Model file for the job. Use its own axes, mm. Give positions to 0.01 mm unless a question says otherwise; leave off trailing zeros. Order: outer loops, then holes, each group sorted by start corner. A loop starts at its lowest first (then second) coordinate and runs counter-clockwise, first axis right, second up. Notation, with made-up numbers: (8, 57.5) -> (20, 57.5) arc R29 ccw to (20, 88.5) -> close; hole circle Ø9 at (24, -10.75). An arc over 180 degrees is marked (long way). Use CSV: the item, a comma, the result in double quotes. Start each with the question number.
1. Wall check: line 1 (Y direction, x = 4, z = -104.5); line 2 (Z direction, x = 14.5, y = 1); line 3 (Z direction, x = 1.5, y = 18). Give the ranges that are in metal, low to high. Write a range as from..to.
2. Cut at A-A on x = 8. List the corners of the cut face in (y, z).
3. Drop flat-ended pins along their axis: pin 1 (4.5 mm diameter, centred on y = 0, z = 45.54, fed in from -X) (3 decimals); pin 2 (8 mm diameter, centred on x = 6.5, y = -4.5, fed in from +Z); pin 3 (6 mm diameter, centred on x = 15, y = 13, fed in from +Z). Give the stop position or say it passes through.
4. Cut at B-B on y = 0. List the corners of the cut face in (x, z), then the cut area to 3 significant figures.
5. Pull direction Y, two halves, no side cores. Call faces 1 (the cylindrical face through (10.14, -18.225, 92.563)), 2 (the cylindrical face through (10.14, 0.11, 48.033)), 3 (the flat face through (0, 0, -17)), 4 (the flat face through (9.86, 2.71, 77.2)): released by +Y, released by -Y, zero draft, split by the parting line, or undercut.
```python
from build123d import *

# Parameters (mm, degrees)
BOSS_EXTRUDE1_DEPTH    = 20
M6_TAPPED_HOLE1_D      = 5
FILLET1_R              = 3
OTW_R_GWINTOWANY_M51_D = 4.2


with BuildPart() as part:
    # Sketch3 → Boss-Extrude1 (new body)
    with BuildSketch(Plane(origin=(0, 0, 0), x_dir=(0, 0, -1), z_dir=(1, 0, 0))):
        Polygon((-62.694317427, 20), (-96.258302674, -20), (130, -20), (130, 20), align=None)
    extrude(amount=BOSS_EXTRUDE1_DEPTH)

    # M6 Tapped Hole1 (through all)
    with Locations(Plane.ZY):
        with Locations((45.535720528, 0), (-104.464279472, 0)):
            Hole(M6_TAPPED_HOLE1_D / 2)

    # Fillet1
    fillet1_edges = [part.edges().sort_by_distance(p)[0] for p in [
        (10, -20, 96.258302674),
    ]]
    fillet(fillet1_edges, radius=FILLET1_R)

    # Otwór gwintowany M51 (through all)
    with Locations(Plane(origin=(20, 0, 0), x_dir=(0, 0, -1), z_dir=(1, 0, 0))):
        with Locations((-71.643866315, 0), (71.643866315, 0)):
            Hole(OTW_R_GWINTOWANY_M51_D / 2)


solid = part.part
```
Verdict:
1,line 1,"-20..-2.5, 2.5..20"
1,line 2,"-130..-106.76, -102.17..-73.49, -69.8..43.24, 47.83..69.8, 73.49..78.64"
1,line 3,"-130..64.37"
2,outline,"(-20, -130) -> (20, -130) -> (20, 62.69) -> (-15.07, 92.12) arc R3 ccw to (-20, 89.82) -> close; hole circle Ø5 at (0, -104.46); hole circle Ø5 at (0, 45.54); hole circle Ø4.2 at (0, -71.64); hole circle Ø4.2 at (0, 71.64)"
3,pin 1,"through"
3,pin 2,"z = 86.61"
3,pin 3,"z = 71.09"
4,outline,"(0, -130) -> (20, -130) -> (20, -106.96) -> (0, -106.96) -> close; (0, -101.96) -> (20, -101.96) -> (20, -73.74) -> (0, -73.74) -> close; (0, -69.54) -> (20, -69.54) -> (20, 43.04) -> (0, 43.04) -> close; (0, 48.04) -> (20, 48.04) -> (20, 69.54) -> (0, 69.54) -> close; (0, 73.74) -> (20, 73.74) -> (20, 79.48) -> (0, 79.48) -> close"
4,area,"3,820 mm^2"
5,face 1,"split by the parting line"
5,face 2,"undercut"
5,face 3,"zero draft"
5,face 4,"released by +Y"
